```python
from build123d import *

# Parameters (mm, degrees)
SKETCH2_R               = 17.7
BOSS_EXTRUDE3_DEPTH     = 3
SKETCH3_R               = 3.1
CUT_EXTRUDE3_DEPTH      = 4
CUT_EXTRUDE3_DEPTH_BACK = 1
SKETCH5_R               = 6.1
BOSS_EXTRUDE4_DEPTH     = 9
SKETCH4_R               = 1.58
CUT_EXTRUDE4_DEPTH      = 13
CUT_EXTRUDE4_DEPTH_BACK = 1
SKETCH6_R               = 3.1
CUT_EXTRUDE5_DEPTH      = 10
SKETCH7_W               = 6.2
SKETCH7_H               = 2.46
BOSS_EXTRUDE5_DEPTH     = 12


with BuildPart() as part:
    # Sketch2 → Boss-Extrude3 (new body)
    with BuildSketch(Plane(origin=(0, 0, 0), x_dir=(-1, 0, 0), z_dir=(0, 1, 0))):
        Circle(SKETCH2_R)
    extrude(amount=BOSS_EXTRUDE3_DEPTH)

    # Sketch3 → Cut-Extrude3 (cut, two sides)
    with BuildSketch(Plane(origin=(0, 0, 0), x_dir=(1, 0, 0), z_dir=(0, 1, 0))) as cut_extrude3_sk:
        Circle(SKETCH3_R)
    extrude(amount=CUT_EXTRUDE3_DEPTH, mode=Mode.SUBTRACT)
    extrude(cut_extrude3_sk.sketch, amount=-CUT_EXTRUDE3_DEPTH_BACK, mode=Mode.SUBTRACT)

    # Sketch5 → Boss-Extrude4 (add)
    with BuildSketch(Plane(origin=(0, 3, 0), x_dir=(1, 0, 0), z_dir=(0, 1, 0))):
        Circle(SKETCH5_R)
    extrude(amount=BOSS_EXTRUDE4_DEPTH)

    # Sketch4 → Cut-Extrude4 (cut, two sides)
    with BuildSketch(Plane(origin=(0, 0, 0), x_dir=(1, 0, 0), z_dir=(0, 1, 0))) as cut_extrude4_sk:
        with Locations((-9, 0)):
            Circle(SKETCH4_R)
        with Locations((9, 0)):
            Circle(SKETCH4_R)
        with Locations((0, 9)):
            Circle(SKETCH4_R)
        with Locations((0, -9)):
            Circle(SKETCH4_R)
    extrude(amount=CUT_EXTRUDE4_DEPTH, mode=Mode.SUBTRACT)
    extrude(cut_extrude4_sk.sketch, amount=-CUT_EXTRUDE4_DEPTH_BACK, mode=Mode.SUBTRACT)

    # Sketch6 → Cut-Extrude5 (cut)
    with BuildSketch(Plane.XZ.offset(-3)):
        Circle(SKETCH6_R)
    extrude(amount=-CUT_EXTRUDE5_DEPTH, mode=Mode.SUBTRACT)

    # Sketch7 → Boss-Extrude5 (add)
    with BuildSketch(Plane.XZ):
        with Locations((0, 1.87)):
            Rectangle(SKETCH7_W, SKETCH7_H)
    extrude(amount=-BOSS_EXTRUDE5_DEPTH)


solid = part.part
```
Input: part model. Units: mm. Frame: model coordinates. A direction names the side the tool comes from. Coordinates: 2 decimals unless noted, no trailing zeros. Loops run counter-clockwise (first coordinate to the right, second up) from the corner with the lowest first, then second, coordinate; pieces in that order, holes last. Notation, with made-up numbers: (86, -13) - (126, -13) arc R18 cw to (126, -5) - close; hole circle Ø9 at (15, 71). An arc over 180 degrees is marked (long way). Answer in a Markdown table with one row per item.
(1) Cut plane A-A on x = 0. Output: boundary loops of the cut face in (y, z), plus the area to 3 significant figures.
Model answer:
| item | result |
|---|---|
| outline | (0, -17.7) - (3, -17.7) - (3, -10.58) - (0, -10.58) - close; (0, -7.42) - (3, -7.42) - (3, -6.1) - (12, -6.1) - (12, -3.1) - (0, -3.1) - close; (0, 0.64) - (12, 0.64) - (12, 6.1) - (3, 6.1) - (3, 7.42) - (0, 7.42) - close; (0, 10.58) - (3, 10.58) - (3, 17.7) - (0, 17.7) - close |
| area | 152 mm² |
(2) Mould query, pull axis Z, two halves, no side actions, for faces 1 (the face through (0, 12, 1)), 2 (the face through (-10.58, 1.48, -0.07)), 3 (the face through (-6.094, 7.437, -0.268)). Classes: pulls with the +Z half, pulls with the -Z half, needs draft (parallel to the pull), parting line crosses it, or undercut.
Model answer:
| item | result |
|---|---|
| face 1 | needs draft |
| face 2 | undercut |
| face 3 | parting line crosses it |
(3) Pin query (flat end, axial travel): P1, Ø5, axis at x = -12, z = 0.5, coming from the +Y side; P2, Ø7, axis at x = 0, z = 0, coming from the -Y side; P3, Ø1.5, axis at y = 3.5, z = 12.5, coming from the -X side; P4, Ø1, axis at x = 0.5, y = 7, coming from the +Z side. Return the tip coordinate at first contact, or that it passes through.
Model answer:
| item | result |
|---|---|
| P1 | stops at y = 3 |
| P2 | stops at y = 0 |
| P3 | stops at x = -13.07 |
| P4 | stops at z = 6.1 |
(4) Set-up query: faces 4 (the face through (4, 0, 0)), 5 (the face through (-8, 3, -4)), 6 (the face through (0, 6, 0.64)). Return all of +Z, -Z, +X, -X, +Y, -Y with unobstructed straight access to the full face (end or side cutting, diameter ignored); none if empty.
Model answer:
| item | result |
|---|---|
| face 4 | +Z, -Z, +X, -X, -Y |
| face 5 | +Y |
| face 6 | +Y, -Y |
(5) Cut plane B-B on z = 0. Output: boundary loops of the cut face in (x, y), plus the area to 3 significant figures.
Model answer:
| item | result |
|---|---|
| outline | (-17.7, 0) - (-10.58, 0) - (-10.58, 3) - (-17.7, 3) - close; (-7.42, 0) - (-3.1, 0) - (-3.1, 12) - (-6.1, 12) - (-6.1, 3) - (-7.42, 3) - close; (3.1, 0) - (7.42, 0) - (7.42, 3) - (6.1, 3) - (6.1, 12) - (3.1, 12) - close; (10.58, 0) - (17.7, 0) - (17.7, 3) - (10.58, 3) - close |
| area | 123 mm² |
(6) Cut plane D-D on z = 9.5. Output: boundary loops of the cut face in (x, y), plus the area to 3 significant figures.
Model answer:
| item | result |
|---|---|
| outline | (-14.93, 0) - (-1.5, 0) - (-1.5, 3) - (-14.93, 3) - close; (1.5, 0) - (14.93, 0) - (14.93, 3) - (1.5, 3) - close |
| area | 80.6 mm² |
(7) Material intervals for L1, parallel to Z at x = 0, y = 1.05; L2, parallel to Z at x = 0, y = 8.25; L3, parallel to Z at x = 9, y = 1.15, sorted ascending. Write a range as from..to.
Model answer:
| item | result |
|---|---|
| L1 | z = -17.7..-10.58, -7.42..-3.1, 0.64..7.42, 10.58..17.7 |
| L2 | z = -6.1..-3.1, 0.64..6.1 |
| L3 | z = -15.24..-1.58, 1.58..15.24 |
(8) Cut plane C-C on y = 1. Output: boundary loops of the cut face in (x, z), plus the area to 3 significant figures.
Model answer:
| item | result |
|---|---|
| outline | circle Ø35.4 at (0, 0); hole circle Ø3.16 at (-9, 0); hole (-3.03, 0.64) arc R3.1 ccw (long way) to (3.03, 0.64) - close; hole circle Ø3.16 at (0, -9); hole circle Ø3.16 at (0, 9); hole circle Ø3.16 at (9, 0) |
| area | 934 mm² |
